```python
from build123d import *

# Parameters (mm, degrees)
F0_W     = 40
F0_H     = 3.3
F1_ANGLE = 270


with BuildPart() as f1:
    # F0 (on Front) → F1 (revolve)
    with BuildSketch(Plane.XZ):
        Polygon((63.284774, 35.914096), (60.584774, 35.914096), (57.116487, 24.914096), (54.353061, 24.914096), (50.884774, 35.914096), (47.934774, 35.914096), (47.934774, 9.714096), (87.934774, 9.714096), (87.934774, 35.914096), (85.384774, 35.914096), (81.916487, 24.914096), (79.153061, 24.914096), (75.684774, 35.914096), (72.984774, 35.914096), (69.516487, 24.914096), (66.753061, 24.914096), align=None)
        with Locations((67.934774, 8.064096)):
            Rectangle(F0_W, F0_H)
    revolve(axis=Axis((67.934774, 0, -5.585904), (-1, 0, 0)), revolution_arc=F1_ANGLE)


solid = f1.part
```
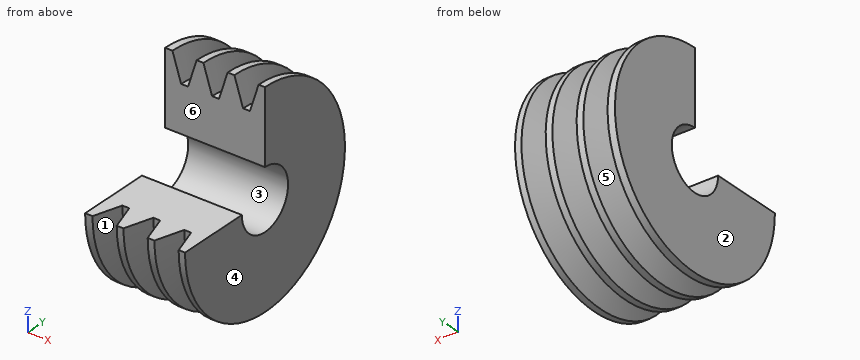
Geometry check sheet. Reference: the model listing, model coordinates, mm. Face numbers are marked on the shaded views. A direction names the side the tool comes from. Coordinates: 2 decimals unless noted, no trailing zeros. Loops run counter-clockwise (first coordinate to the right, second up) from the corner with the lowest first, then second, coordinate; pieces in that order, holes last.
Item 1: Thickness scan on line 1 (X direction, y = 34.5, z = -3.5); line 2 (X direction, y = 33, z = -18); line 3 (Y direction, x = 55.5, z = -29). Record the ranges inside material, lowest first.
Item 2: Go/stop test with a flat-tipped pin: pin 1 Ø23.5 at (x, y) = (67.5, -21) entering from +Z. Record where the tip stops, or that it passes through.
Item 3: Access from +Z, -Z, +X, -X, +Y, -Y to the whole of each face (thin tool, end or side, straight path). Record for the marked faces 4, 5 and 6.
Item 4: Sectioned sample at D-D, the plane x = 78. Record the boundary of the cut face in (y, z).
Item 5: Sectioned sample at B-B, the plane x = 56. Record the boundary of the cut face in (y, z).
Item 6: Sectioned sample at A-A, the plane z = -39. Count the separate pieces of the cut face and the enclosed holes in it, then the cut area to 3 significant figures.
Item 7: Release check for a two-part mould opening along Y. For the marked faces 1, 2 and 3 record: released by +Y, released by -Y, zero draft, split by the parting line, or undercut.
Check result:
1. line 1: x = 47.93 to 53.07, 58.4 to 65.47, 70.8 to 77.87, 83.2 to 87.93
1. line 2: x = 47.93 to 52.85, 58.62 to 65.25, 71.02 to 77.65, 83.42 to 87.93
1. line 3: y = -19.55 to 19.55
2. pin 1: stops at z = -5.59
3. face 4: +Z, -Z, +X, +Y, -Y
3. face 5: none
3. face 6: +Z, +X, -X, -Y
4. outline: (-34.16, -5.59) arc R34.16 ccw (long way) to (0, 28.57) - (0, 6.41) arc R12 cw (long way) to (-12, -5.59) - close
5. outline: (-30.5, -5.59) arc R30.5 ccw (long way) to (0, 24.91) - (0, 6.41) arc R12 cw (long way) to (-12, -5.59) - close
6. separate pieces: 4
6. enclosed holes: 0
6. area: 1,030 mm2
7. face 1: split by the parting line
7. face 2: zero draft
7. face 3: undercut
